The listing builds one solid part. Answer for the finished solid, in the listing's coordinates (mm). Face numbers are marked on the shaded views. A direction names the side the tool comes from. Give positions to 0.01 mm unless a question says otherwise; leave off trailing zeros. Order: outer loops, then holes, each group sorted by start corner. A loop starts at its lowest first (then second) coordinate and runs counter-clockwise, first axis right, second up. Notation, with made-up numbers: (-27, 53) - (-9, 53) arc R23 cw to (-9, 62) - close; hole circle Ø2 at (9.25, 19.5). An arc over 180 degrees is marked (long way). Answer in a Markdown table with one row per item. Add a question column.
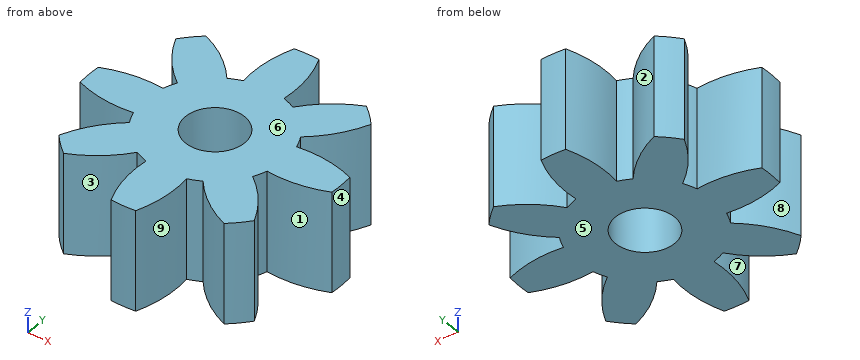
Autodesk Inventor part; units mm, degrees
ref_plane "Work Plane2" through (0, 0, 2) normal (0, 0, 1) x (1, 0, 0)
ref_plane "Work Plane8" through (0, 0, 0) normal (0.9238795, 0.3826834, 0) x (0, 0, 1)
ref_plane "Work Plane9" through (0, 0, 0) normal (1, 0, 0) x (0, 1, 0)
sketch "Sketch1" plane through (0, 0, 0) normal (0, 0, 1) x (1, 0, 0)
  circle A0 centre (0, 0) radius 4.9765
  dimension "d0" = 9.953
extrude "Extrusion1" add sketch "Sketch1" along normal blind 4
ref_plane "Work Plane2" through (0, 0, 2) normal (0, 0, 1) x (1, 0, 0)
sketch "Sketch2" plane through (0, 0, 0) normal (0, 0, -1) x (-1, 0, 0)
  circle A0 centre (0, 0) radius 4.9765
  circle A1 centre (0, 0) radius 4
  dimension "d3" = 8
surface extrude "節圓直徑" sketch "Sketch2" against normal through all shown no curves A1
ref_plane "Work Plane8" through (0, 0, 0) normal (0.9238795, 0.3826834, 0) x (0, 0, 1)
ref_plane "Work Plane9" through (0, 0, 0) normal (1, 0, 0) x (0, 1, 0)
spur gear teeth "正齒輪" teeth 8 pitch diameter 8 tip diameter 9.953 root diameter 5.5 face width 4 start plane through (0, 0, 0) normal (0, 0, -1) x (-1, 0, 0)
sketch "草圖3" plane through (0, 0, 4) normal (0, 0, 1) x (1, 0, 0)
  circle A0 centre (0, 0) radius 1.175
  dimension "d49" = 2.35
extrude "擠出2" cut sketch "草圖3" against normal up to next
equation "\"d0\" = da_da"
equation "\"d1\" = da_b"
equation "\"d3\" = da_d"
equation "\"d16\" = da_aw"
equation "\"d43\" = da_aw"
equation "\"d46\" = da_aw"
properties part number "正齒輪1" material "Steel"
(1) The mould has two halves that part along X. Classify the marked faces 6, 7, 8 and 9: +X half, -X half, draft (parallel to the pull), parting line (faces both ways), or undercut.
(2) Find section A-A, the plane y = 0. Write down the section's boundary in (x, z) (1 decimal), plus the area to 3 significant figures.
(3) For the marked faces 1, 2, 3, 4 and 5, determine the directions among +Z, -Z, +X, -X, +Y, -Y from which every point of the face is accessible in a straight line to the end or side of a thin tool.
(4) Straight lines are drawn through the part: line 1 (Y direction, x = 3.75, z = 1.6); line 2 (Y direction, x = 0, z = 1.2) (1 decimal); line 3 (X direction, y = 3, z = 3.2). For each, find the intervals that lie inside material, in ascending order.
(5) This flat-tipped pin is pushed along its axis until it touches: P1, Ø2.5, axis at x = 0, y = 0, coming from the -Z side. Where does it stop, or does it pass through?
(6) Find section D-D, the plane x = 3. Write down the section's boundary in (y, z), plus the area to 3 significant figures.
Answer key:
| question | item | result |
|---|---|---|
| 1 | face 6 | draft |
| 1 | face 7 | undercut |
| 1 | face 8 | -X half |
| 1 | face 9 | undercut |
| 2 | outline | (-5, 0) - (-1.2, 0) - (-1.2, 4) - (-5, 4) - close; (1.2, 0) - (5, 0) - (5, 4) - (1.2, 4) - close |
| 2 | area | 30.4 mm² |
| 3 | face 1 | +Z, -Z |
| 3 | face 2 | +Z, -Z, +Y |
| 3 | face 3 | +Z, -Z, -Y |
| 3 | face 4 | +Z, -Z, +X |
| 3 | face 5 | -Z, +X, -X, +Y, -Y |
| 4 | line 1 | -3.27 to -2.94, -0.8 to 0.8, 2.94 to 3.27 |
| 4 | line 2 | -5 to -1.2, 1.2 to 5 |
| 4 | line 3 | -3.78 to -1.83, -0.83 to 0.83, 1.83 to 3.78 |
| 5 | P1 | z = 0 |
| 6 | outline | (-3.78, 0) - (-1.83, 0) - (-1.83, 4) - (-3.78, 4) - close; (-0.83, 0) - (0.83, 0) - (0.83, 4) - (-0.83, 4) - close; (1.83, 0) - (3.78, 0) - (3.78, 4) - (1.83, 4) - close |
| 6 | area | 22.2 mm² |
